CAD build for the part. Positions are in the model's coordinates, mm. Coordinates: 2 decimals unless noted, no trailing zeros. Loops run counter-clockwise (first coordinate to the right, second up) from the corner with the lowest first, then second, coordinate; pieces in that order, holes last. Notation, with made-up numbers: (2, 16) -> (43, 16) arc R25 cw to (43, 50) -> close; hole circle Ø3 at (-36, -2). An arc over 180 degrees is marked (long way). Answer as CSV lines item,"result". Start each with the question number.
```python
from build123d import *

# Parameters (mm, degrees)
SKETCH1_R           = 1000
BOSS_EXTRUDE2_DEPTH = 1
DOME1_FACE_RADIUS   = 1000
DOME1_HEIGHT        = 1000
CUT_EXTRUDE1_START  = -300
SKETCH2_R           = 1000
CUT_EXTRUDE1_DEPTH  = 300
SKETCH4_R           = 1000
CUT_EXTRUDE2_DEPTH  = 660


with BuildPart() as part:
    # Sketch1 → Boss-Extrude2 (new body)
    with BuildSketch(Plane.XY):
        Circle(SKETCH1_R)
    extrude(amount=BOSS_EXTRUDE2_DEPTH)

    # Dome1: a dome of height H over a round flat face of radius A is a cap of a sphere of radius (A * A + H * H) / (2 * H)
    dome1_r = (DOME1_FACE_RADIUS * DOME1_FACE_RADIUS + DOME1_HEIGHT * DOME1_HEIGHT) / (2 * DOME1_HEIGHT)
    dome1_base = Plane((0, 0, 1), z_dir=(0, 0, 1))
    with Locations(dome1_base.offset(DOME1_HEIGHT - dome1_r)):
        dome1_ball = Sphere(dome1_r, mode=Mode.PRIVATE)
    add(split(dome1_ball, bisect_by=dome1_base, keep=Keep.TOP, mode=Mode.PRIVATE))

    # Sketch2 → Cut-Extrude1 (cut)
    with BuildSketch(Plane.XY.offset(1001).offset(CUT_EXTRUDE1_START)):
        Circle(SKETCH2_R)
    extrude(amount=CUT_EXTRUDE1_DEPTH, mode=Mode.SUBTRACT)

    # Sketch4 → Cut-Extrude2 (cut)
    with BuildSketch(Plane(origin=(0, 0, 0), x_dir=(-1, 0, 0), z_dir=(0, 0, -1))):
        Circle(SKETCH4_R)
    extrude(amount=-CUT_EXTRUDE2_DEPTH, mode=Mode.SUBTRACT)


solid = part.part
```
Q1. Saw through at A-A (y = -580.5). List the corners of the cut face in (x, z).
Q2. Probe probe 1 along X at (y, z) = (309, 675); probe 2 along Y at (x, z) = (83, 692); probe 3 along Y at (x, z) = (-394, 689.5). List the from-to ranges inside material, lowest first. Write a range as from..to.
Q3. Pin check, flat tips, straight feed: pin 1 Ø12 at (y, z) = (-425.5, 685.5) entering from +X; pin 2 Ø8 at (y, z) = (166, 677) entering from -X; pin 3 Ø6 at (x, z) = (280.5, 678.5) entering from -Y. Stop position of each tip, or through.
Q4. Saw through at C-C (z = 682.5). List the corners of the cut face in (x, y), and give its area (3 significant figures).
Q5. Saw through at B-B (x = 526.5). List the corners of the cut face in (y, z).
Ans:
1,outline,"(-478.27, 660) -> (478.27, 660) arc R814.26 ccw to (415.96, 701) -> (-415.96, 701) arc R814.26 ccw to start"
2,probe 1,"x = -671..671"
2,probe 2,"y = -718.07..718.07"
2,probe 3,"y = -608.88..608.88"
3,pin 1,"stops at x = 600.04"
3,pin 2,"stops at x = -721.82"
3,pin 3,"stops at y = -683.16"
4,outline,"circle Ø1463.64 at (0, 0)"
4,area,"1,680,000 mm²"
5,outline,"(-537.14, 660) -> (537.14, 660) arc R850.18 ccw to (482.49, 701) -> (-482.49, 701) arc R850.18 ccw to start"
